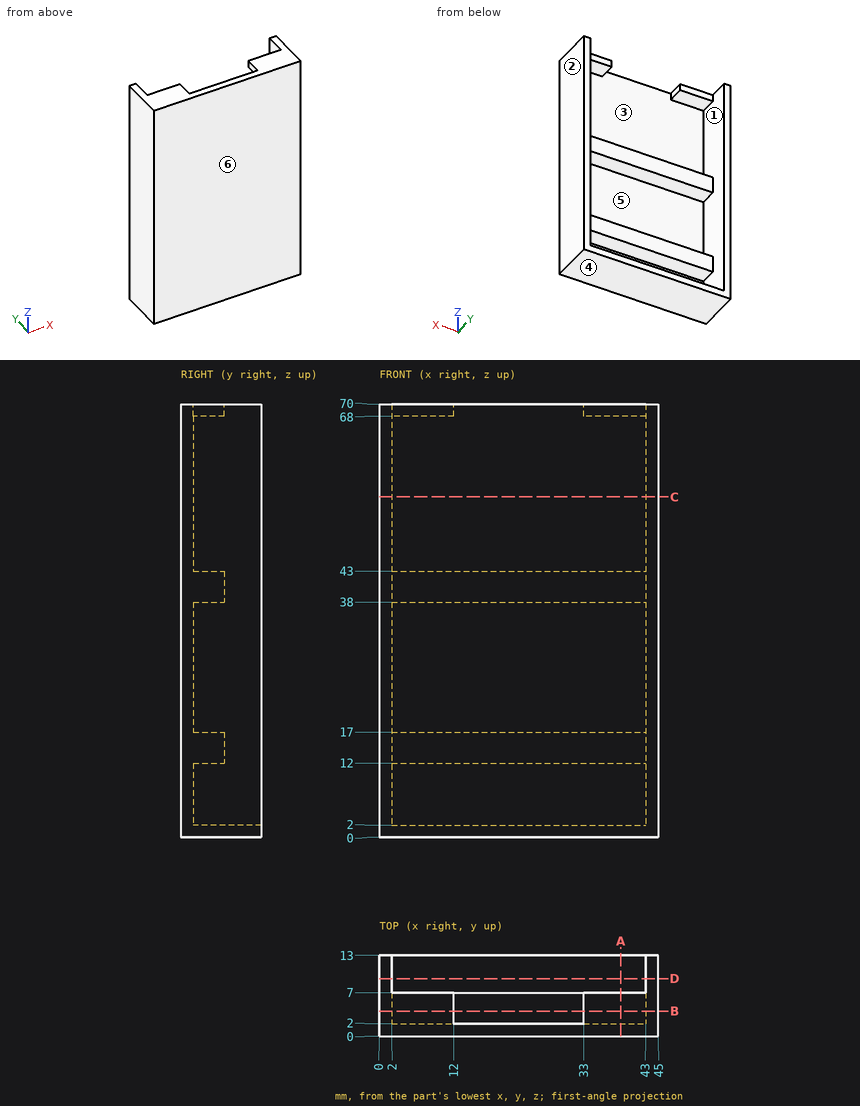
Input: dimensioned drawing with shaded views. Units: mm. Origin: part minimum x, y, z. A direction names the side the tool comes from. Coordinates: 2 decimals unless noted, no trailing zeros. Order: outer loops, then holes, each group sorted by start corner. A loop starts at its lowest first (then second) coordinate and runs counter-clockwise, first axis right, second up.
1. Draft query along Z for the marked faces 1, 2, 3 and 4. Return one class per face: +Z half, -Z half, draft (parallel to the pull), parting line (faces both ways), or undercut.
Checked values:
face 1: undercut
face 2: draft
face 3: undercut
face 4: -Z half
2. Cut plane B-B, the plane y = 4. Return loops of the section in (x, z).
Checked values:
outline: (0, 0) - (45, 0) - (45, 70) - (33, 70) - (33, 68) - (43, 68) - (43, 43) - (2, 43) - (2, 68) - (12, 68) - (12, 70) - (0, 70) - close; hole (2, 2) - (43, 2) - (43, 12) - (2, 12) - close; hole (2, 17) - (43, 17) - (43, 38) - (2, 38) - close
3. Access query for the marked faces 5 and 6. Directions: +Z, -Z, +X, -X, +Y, -Y. A direction counts if a zero-diameter tool reaches every point of the face in a straight line with its end or side. Return the directions, or none.
Checked values:
face 5: +Y
face 6: +Z, -Z, +X, -X, -Y
4. Cut plane D-D, the plane y = 9.25. Return loops of the section in (x, z), plus the area to 3 significant figures.
Checked values:
outline: (0, 0) - (45, 0) - (45, 70) - (43, 70) - (43, 2) - (2, 2) - (2, 70) - (0, 70) - close
area: 362 mm2
5. Cut plane C-C, the plane z = 55. Return loops of the section in (x, y), plus the area to 3 significant figures.
Checked values:
outline: (0, 0) - (45, 0) - (45, 13) - (43, 13) - (43, 2) - (2, 2) - (2, 13) - (0, 13) - close
area: 134 mm2
6. Ray query, line 1 along Z through (x, y) = (18, 4); line 2 along X through (y, z) = (5.25, 19); line 3 along Z through (x, y) = (11.5, 4.75). Return the intervals inside material, ascending.
Checked values:
line 1: z = 0 to 2, 12 to 17, 38 to 43
line 2: x = 0 to 2, 43 to 45
line 3: z = 0 to 2, 12 to 17, 38 to 43, 68 to 70
7. Contact query for flat-ended pins moving along their axis: P1, Ø2, axis at x = 18, y = 11, coming from the +Z side; P2, Ø8, axis at x = 23, z = 57, coming from the +Y side; P3, Ø4, axis at x = 19.5, z = 41, coming from the +Y side. Output: stop coordinate, or through.
Checked values:
P1: stops at z = 2
P2: stops at y = 2
P3: stops at y = 7
8. Cut plane A-A, the plane x = 39. Return loops of the section in (y, z), plus the area to 3 significant figures.
Checked values:
outline: (0, 0) - (13, 0) - (13, 2) - (2, 2) - (2, 12) - (7, 12) - (7, 17) - (2, 17) - (2, 38) - (7, 38) - (7, 43) - (2, 43) - (2, 68) - (7, 68) - (7, 70) - (0, 70) - close
area: 222 mm2
